Part model, mm, in its own coordinate system. A direction names the side the tool comes from. Round coordinates to 2 decimals unless told otherwise and drop trailing zeros. Order: outer loops, then holes, each group sorted by start corner. A loop starts at its lowest first (then second) coordinate and runs counter-clockwise, first axis right, second up. Notation, with made-up numbers: (34.5, -7) -> (38.5, -7) arc R32 cw to (38.5, 31) -> close; hole circle Ø10 at (-33, -23). An arc over 180 degrees is marked (long way). Use CSV: the item, a comma, the result in double quotes.
```python
from build123d import *

# Parameters (mm, degrees)
F0_R     = 12.7
F0_R_2   = 4.7625
F1_DEPTH = 3.175
F2_R     = 15.875
F2_R_2   = 4.7625
F3_DEPTH = 4.445
F4_R     = 15.875
F4_R_2   = 12.7
F5_DEPTH = 25.4
F6_SIZE  = 0.762
F7_SIZE  = 0.381


with BuildPart() as f1:
    # F0 (on Front) → F1 (new body)
    with BuildSketch(Plane.XZ):
        Circle(F0_R)
        Circle(F0_R_2, mode=Mode.SUBTRACT)
    extrude(amount=-F1_DEPTH)

    # F2 (on Front) → F3 (join)
    with BuildSketch(Plane.XZ):
        Circle(F2_R)
        Circle(F2_R_2, mode=Mode.SUBTRACT)
    extrude(amount=F3_DEPTH)

    # F4 (on Front) → F5 (join)
    with BuildSketch(Plane.XZ):
        Circle(F4_R)
        Circle(F4_R_2, mode=Mode.SUBTRACT)
    extrude(amount=F5_DEPTH)

    # F6
    f6_edges = [f1.edges().sort_by_distance(p)[0] for p in [
        (-12.7, -25.4, 0),
        (-15.875, -25.4, 0),
        (-4.7625, -4.445, 0),
        (-12.7, 3.175, 0),
        (-4.7625, 3.175, 0),
    ]]
    chamfer(f6_edges, length=F6_SIZE)

    # F7
    f7_edges = [f1.edges().sort_by_distance(p)[0] for p in [
        (-15.875, 0, 0),
    ]]
    chamfer(f7_edges, length=F7_SIZE)


solid = f1.part
```
(1) Drop flat-ended pins along their axis: P1, Ø1.5, axis at x = -11.5, z = -8, coming from the +Y side; P2, Ø4, axis at x = 6.5, y = -21.5, coming from the +Z side; P3, Ø3, axis at x = -11.5, z = 3.5, coming from the -Y side; P4, Ø5, axis at x = 12, y = -14.5, coming from the +Z side. Give the stop position or say it passes through.
Reply:
P1,"y = 0"
P2,"z = 15.22"
P3,"y = -25.4"
P4,"z = 12.72"
(2) Cut at C-C, the plane y = 0.75. Give the cut face in (x, z) (1 decimal), then the cut area to 3 significant figures.
Reply:
outline,"circle Ø25.4 at (0, 0); hole circle Ø9.5 at (0, 0)"
area,"435 mm2"
(3) Probe probe 1 along Z at (x, y) = (0, -10) (3 decimals); probe 2 along Z at (x, y) = (0, 0.25); probe 3 along X at (y, z) = (-18.5, 3.5). List the from-to ranges inside material, lowest first. Write a range as [from, to].
Reply:
probe 1,"[-15.875, -12.7], [12.7, 15.875]"
probe 2,"[-12.7, -4.76], [4.76, 12.7]"
probe 3,"[-15.48, -12.21], [12.21, 15.48]"
(4) Pull direction Z, two halves, no side cores. Call faces 4 (the face through (5, -4.445, -3)), 5 (the face through (-1, 0, 13)), 6 (the face through (-3.441, -12.34, -15.497)): released by +Z, released by -Z, zero draft, split by the parting line, or undercut.
Reply:
face 4,"undercut"
face 5,"zero draft"
face 6,"split by the parting line"
(5) Cut at A-A, the plane z = 0. Give the cut face in (x, y) (1 decimal).
Reply:
outline,"(-15.9, -24.6) -> (-15.1, -25.4) -> (-13.5, -25.4) -> (-12.7, -24.6) -> (-12.7, -4.4) -> (-5.5, -4.4) -> (-4.8, -3.7) -> (-4.8, 2.4) -> (-5.5, 3.2) -> (-11.9, 3.2) -> (-12.7, 2.4) -> (-12.7, 0) -> (-15.5, 0) -> (-15.9, -0.4) -> close; (4.8, -3.7) -> (5.5, -4.4) -> (12.7, -4.4) -> (12.7, -24.6) -> (13.5, -25.4) -> (15.1, -25.4) -> (15.9, -24.6) -> (15.9, -0.4) -> (15.5, 0) -> (12.7, 0) -> (12.7, 2.4) -> (11.9, 3.2) -> (5.5, 3.2) -> (4.8, 2.4) -> close"
(6) Which spindle directions (+Z, -Z, +X, -X, +Y, -Y) get a long thin tool onto all of the face, cutting with end or side? Do faces 1 (the face through (-2.75, -14.4, -12.4)), 2 (the face through (-2.75, 1.19, -12.4)), 3 (the face through (-3.78, -0.59, -2.9)). Say none if no direction does.
Reply:
face 1,"-Y"
face 2,"+Y"
face 3,"+Y, -Y"
(7) Cut at B-B, the plane x = 0. Give the cut face in (y, z) (1 decimal).
Reply:
outline,"(-25.4, -15.1) -> (-24.6, -15.9) -> (-0.4, -15.9) -> (0, -15.5) -> (0, -12.7) -> (2.4, -12.7) -> (3.2, -11.9) -> (3.2, -5.5) -> (2.4, -4.8) -> (-3.7, -4.8) -> (-4.4, -5.5) -> (-4.4, -12.7) -> (-24.6, -12.7) -> (-25.4, -13.5) -> close; (-25.4, 13.5) -> (-24.6, 12.7) -> (-4.4, 12.7) -> (-4.4, 5.5) -> (-3.7, 4.8) -> (2.4, 4.8) -> (3.2, 5.5) -> (3.2, 11.9) -> (2.4, 12.7) -> (0, 12.7) -> (0, 15.5) -> (-0.4, 15.9) -> (-24.6, 15.9) -> (-25.4, 15.1) -> close"
